Geometry: final body of the model. Coordinates: model frame, mm. Round coordinates to 2 decimals unless told otherwise and drop trailing zeros. Loops run counter-clockwise (first coordinate to the right, second up) from the corner with the lowest first, then second, coordinate; pieces in that order, holes last. Notation, with made-up numbers: M 18,-23 L 56,-23 A27 cw 56,1 Z; hole C 58,1.25 d1. An arc over 180 degrees is marked long. Return JSON: item names as keys, results as strings.
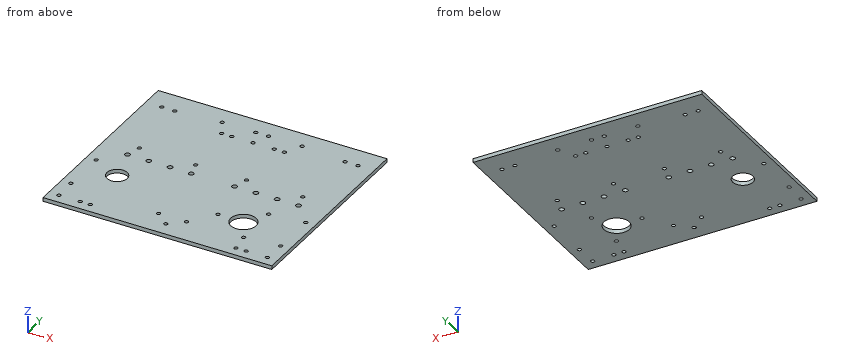
from build123d import *

# Parameters (mm, degrees)
SKETCH_R      = 1.5
SKETCH_R_2    = 2
PAD_DEPTH     = 3
SKETCH001_R   = 8
SKETCH001_R_2 = 1.5
SKETCH001_R_3 = 10
POCKET_DEPTH  = 3.001


with BuildPart() as part:
    # Sketch → Pad (new body)
    with BuildSketch(Plane.XY):
        with BuildLine():
            Line((0, 13.7), (0, 160))
            Line((0, 160), (90, 160))
            Line((90, 160), (90, 17.4))
            Line((90, 17.4), (90, 13.2))
            ThreePointArc((90, 13.2), (88.5, 11.7), (90, 10.2))
            Line((90, 6), (90, 10.2))
            Line((90, 6), (90, 0))
            Line((90, 0), (13.7, 0))
            Line((0, 0), (13.7, 0))
            Line((0, 13.7), (0, 0))
        make_face()
        with Locations((24.7, 8)):
            Circle(SKETCH_R, mode=Mode.SUBTRACT)
        with Locations((32.7, 8)):
            Circle(SKETCH_R, mode=Mode.SUBTRACT)
        with Locations((79, 21)):
            Circle(SKETCH_R, mode=Mode.SUBTRACT)
        with Locations((22.74, 77.15)):
            Circle(SKETCH_R_2, mode=Mode.SUBTRACT)
        with Locations((39.48, 77.15)):
            Circle(SKETCH_R_2, mode=Mode.SUBTRACT)
        with Locations((56.22, 77.15)):
            Circle(SKETCH_R_2, mode=Mode.SUBTRACT)
        with Locations((72.96, 77.15)):
            Circle(SKETCH_R_2, mode=Mode.SUBTRACT)
        with Locations((25.7, 88.45)):
            Circle(SKETCH_R, mode=Mode.SUBTRACT)
        with Locations((70, 88.45)):
            Circle(SKETCH_R, mode=Mode.SUBTRACT)
        with Locations((8, 8)):
            Circle(SKETCH_R, mode=Mode.SUBTRACT)
        with Locations((7.5, 60.5)):
            Circle(SKETCH_R, mode=Mode.SUBTRACT)
        with Locations((7.5, 25.5)):
            Circle(SKETCH_R, mode=Mode.SUBTRACT)
        with Locations((85, 145.5)):
            Circle(SKETCH_R, mode=Mode.SUBTRACT)
        with Locations((58.5, 145.5)):
            Circle(SKETCH_R, mode=Mode.SUBTRACT)
        with Locations((12.8, 142.4)):
            Circle(SKETCH_R, mode=Mode.SUBTRACT)
        with Locations((23, 142.4)):
            Circle(SKETCH_R, mode=Mode.SUBTRACT)
    pad = extrude(amount=PAD_DEPTH)

    # Mirrored: Pad across face of Pad
    add(pad.mirror(Plane(origin=(90, 88.7, 1.5), x_dir=(0, 1, 0), z_dir=(1, 0, 0))))

    # Sketch001 → Pocket (cut, through all)
    with BuildSketch(Plane.XY.offset(3)):
        with Locations((30, 50)):
            Circle(SKETCH001_R)
        with Locations((90, 132.8)):
            Circle(SKETCH001_R_2)
        with Locations((106.7, 132.8)):
            Circle(SKETCH001_R_2)
        with Locations((114.7, 132.8)):
            Circle(SKETCH001_R_2)
        with Locations((73.3, 132.8)):
            Circle(SKETCH001_R_2)
        with Locations((65.3, 132.8)):
            Circle(SKETCH001_R_2)
        with Locations((135, 40)):
            Circle(SKETCH001_R_3)
        with Locations((115, 40)):
            Circle(SKETCH001_R_2)
        with Locations((145, 57.320508)):
            Circle(SKETCH001_R_2)
        with Locations((145, 22.679492)):
            Circle(SKETCH001_R_2)
    extrude(amount=-POCKET_DEPTH, mode=Mode.SUBTRACT)


solid = part.part
Q1. Section query A-A (y = 44). Output: boundary loops of the cut face in (x, z), plus the area to 3 significant figures.
Determined:
{"outline": "M 0,0 L 24.71,0 L 24.71,3 L 0,3 Z; M 35.29,0 L 125.83,0 L 125.83,3 L 35.29,3 Z; M 144.17,0 L 180,0 L 180,3 L 144.17,3 Z", "area": "453 mm^2"}
Q2. Material intervals for L1, parallel to Y at x = 107.04, z = 1.8; L2, parallel to X at y = 20.5, z = 1.3; L3, parallel to Y at x = 154.3, z = 0.9, sorted ascending.
Determined:
{"L1": "y = 0 to 75.15, 79.15 to 131.34, 134.26 to 160", "L2": "x = 0 to 77.59, 80.41 to 99.59, 102.41 to 180", "L3": "y = 0 to 6.88, 9.12 to 86.95, 89.95 to 160"}
Q3. Section query B-B (z = 0.9). State how many separate pieces and enclosed holes the cut face has, plus the area to 3 significant figures.
Determined:
{"separate pieces": "1", "enclosed holes": "43", "area": "28,000 mm^2"}
